Input: part model. Units: mm. Frame: model coordinates. Face numbers are marked on the shaded views. A direction names the side the tool comes from. Give positions to 0.01 mm unless a question says otherwise; leave off trailing zeros. Loops run counter-clockwise (first coordinate to the right, second up) from the corner with the lowest first, then second, coordinate; pieces in that order, holes last. Notation, with made-up numbers: M 12.25,27 L 18.25,27 A25 cw 18.25,45 Z; hole C 68.25,-17.5 d7. An arc over 180 degrees is marked long. Return JSON: item names as keys, results as strings. Group by question number.
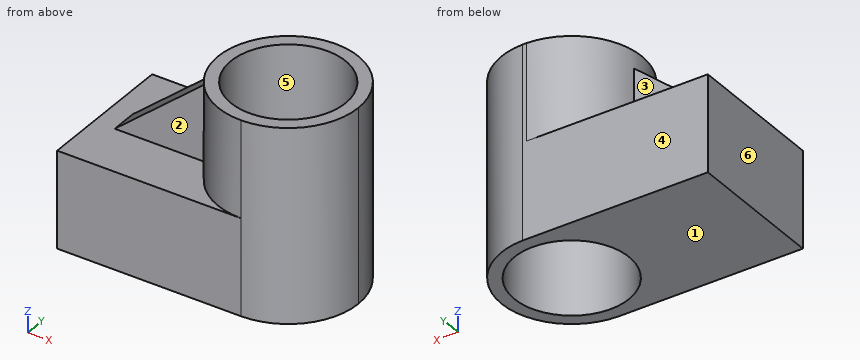
```python
from build123d import *

# Parameters (mm, degrees)
F1_DEPTH = 25.4
F0_R     = 15.0505482929
F2_DEPTH = 50.8
F4_DEPTH = 20.828
F6_DEPTH = 25.4


with BuildPart() as f1:
    # F0 (on Top) → F1 (new body)
    with BuildSketch(Plane.XY):
        with BuildLine():
            Line((-30.0037506968, -18.4360407293), (18.2052805233, -18.4092394559))
            ThreePointArc((18.2052805233, -18.4092394559), (-0.2123373289, -0.2616045695), (17.6821201623, 18.4020952356))
            Line((17.6821201623, 18.4020952356), (-30.0037506968, 18.4020952356))
            Line((-30.0037506968, 18.4020952356), (-30.0037506968, -18.4360407293))
        make_face()
    extrude(amount=F1_DEPTH)

    # F0 (on Top) → F2 (join)
    with BuildSketch(Plane.XY):
        with BuildLine():
            ThreePointArc((18.2052805233, -18.4092394559), (31.2159640874, -13.0136811535), (36.6042884127, 0))
            ThreePointArc((36.6042884127, 0), (31.3924469958, 12.8346722592), (18.7079720616, 18.4020952356))
            Line((18.7079720616, 18.4020952356), (17.6821201623, 18.4020952356))
            ThreePointArc((17.6821201623, 18.4020952356), (-0.2123373289, -0.2616045695), (18.2052805233, -18.4092394559))
        make_face()
        with Locations((18.1950461119, 0)):
            Circle(F0_R, mode=Mode.SUBTRACT)
    extrude(amount=F2_DEPTH)

    # F3 (on face) → F4 (join)
    with BuildSketch(Plane.XY.offset(25.4)):
        with BuildLine():
            ThreePointArc((0, -2.8000891188), (-0.2141961888, 0), (0, 2.8000891188))
            Line((0, 2.8000891188), (-24.5482716709, 2.8000891188))
            Line((-24.5482716709, 2.8000891188), (-24.5482716709, -4.1717705317))
            Line((-24.5482716709, -4.1717705317), (0, -4.1717705317))
            Line((0, -4.1717705317), (0, -2.8000891188))
        make_face()
    extrude(amount=F4_DEPTH)

    # F5 (on face) → F6 (cut)
    with BuildSketch(Plane.XZ.offset(4.1717705317)):
        Polygon((-24.5482716709, 25.4), (0, 46.228), (-24.5482716709, 46.228), align=None)
    extrude(amount=-F6_DEPTH, mode=Mode.SUBTRACT)


solid = f1.part
```
Item 1: Material intervals for line 1 (Z direction, x = -10, y = 15); line 2 (Y direction, x = -1.5, z = 11); line 3 (Y direction, x = -16, z = 31), sorted ascending. Write a range as from..to.
Item 2: Reachability of the marked faces 1, 2 and 3 from +Z, -Z, +X, -X, +Y, -Y: full face, straight path, thin tool, end or side. Return the list, or none.
Item 3: Section D-D, the plane z = 39.5. Return loops of the section in (x, y), then the cut area to 3 significant figures.
Item 4: First-contact query: pin 1 Ø6 at (y, z) = (9.5, 42) entering from -X; pin 2 Ø18 at (x, y) = (18.2, 0) entering from -Z; pin 3 Ø10 at (y, z) = (-4, 32.5) entering from -X; pin 4 Ø23 at (x, z) = (-18.5, 35.5) entering from -Y. Flat tips, straight axial feed; report the tip coordinate or a pass-through.
Item 5: Section B-B, the plane x = 32. Return loops of the section in (y, z).
Item 6: Section C-C, the plane y = 9. Return loops of the section in (x, z).
Item 7: Pull-direction query (X, two-part tool) for the marked faces 4, 5 and 6; classes: pulls with the +X half, pulls with the -X half, needs draft (parallel to the pull), parting line crosses it, or undercut.
Item 8: Section A-A, the plane z = 23. Return loops of the section in (x, y), then the cut area to 3 significant figures.
Answer below:
{
 "1": {"line 1": "0..25.4", "line 2": "-18.42..18.4", "line 3": "-4.17..2.8"},
 "2": {"face 1": "-Z, +X, -X, +Y, -Y", "face 2": "+Z, -X, -Y", "face 3": "+Z, -X, +Y"},
 "3": {"outline": "M -7.93,-4.17 L 0,-4.17 L 0,-2.8 A18.41 ccw long 18.71,18.4 L 17.68,18.4 A18.41 ccw 0,2.8 L -7.93,2.8 Z; hole C 18.2,0 d30.1", "area": "408 mm^2"},
 "4": {"pin 1": "x = 0.97", "pin 2": "through", "pin 3": "x = -22.07", "pin 4": "y = -18.43"},
 "5": {"outline": "M -12.18,0 L -6,0 L -6,50.8 L -12.18,50.8 Z; M 6,0 L 12.18,0 L 12.18,50.8 L 6,50.8 Z"},
 "6": {"outline": "M -30,0 L 6.13,0 L 6.13,50.8 L 2.14,50.8 L 2.14,25.4 L -30,25.4 Z; M 30.26,0 L 34.25,0 L 34.25,50.8 L 30.26,50.8 Z"},
 "7": {"face 4": "needs draft", "face 5": "undercut", "face 6": "pulls with the -X half"},
 "8": {"outline": "M -30,-18.44 L 18.21,-18.41 A18.41 ccw 18.71,18.4 L -30,18.4 Z; hole C 18.2,0 d30.1", "area": "1,600 mm^2"}
}
